For this review, use the dimensioned drawing (mm, ordinates from the lowest corner) and the shaded views. A direction names the side the tool comes from. Round coordinates to 2 decimals unless told otherwise and drop trailing zeros. Loops run counter-clockwise (first coordinate to the right, second up) from the corner with the lowest first, then second, coordinate; pieces in that order, holes last. Notation, with made-up numbers: M 65,44 L 100,44 A8 ccw 100,56 Z; hole C 31.25,-36.75 d8. An arc over 180 degrees is marked long. Answer as a JSON object with one key per item and string values. Group by question number.
Item 1: Consider section A-A (x = 21.5). Give the boundary of the cut face in (y, z), and give its area (3 significant figures).
Item 2: Tool access review of the marked faces 5 and 6: name each direction out of +Z, -Z, +X, -X, +Y, -Y from which nothing blocks a thin tool from reaching the whole face with its end or side.
Item 3: To check wall thickness, follow line 1 (X direction, y = 5.25, z = 36); line 2 (X direction, y = 9, z = 21.5); line 3 (X direction, y = 8.5, z = 35). State the ranges of each line that lie inside material, in increasing order.
Item 4: Consider section B-B (z = 28). Give the boundary of the cut face in (x, y).
Item 5: The part is to be moulded in two halves that separate along X. For the marked faces 1, 2, 3 and 4, say which applies: +X half, -X half, draft (parallel to the pull), parting line (faces both ways), or undercut.
Item 6: Insertion check: P1, Ø4, axis at x = 4, z = 36, coming from the +Y side. The pin has a flat end and moves straight along its axis. Give the tip position at first contact, or say it passes through.
Item 7: Consider section D-D (x = 36). Give the boundary of the cut face in (y, z), and give its area (3 significant figures).
Item 8: Consider section C-C (y = 11.5). Give the boundary of the cut face in (x, z).
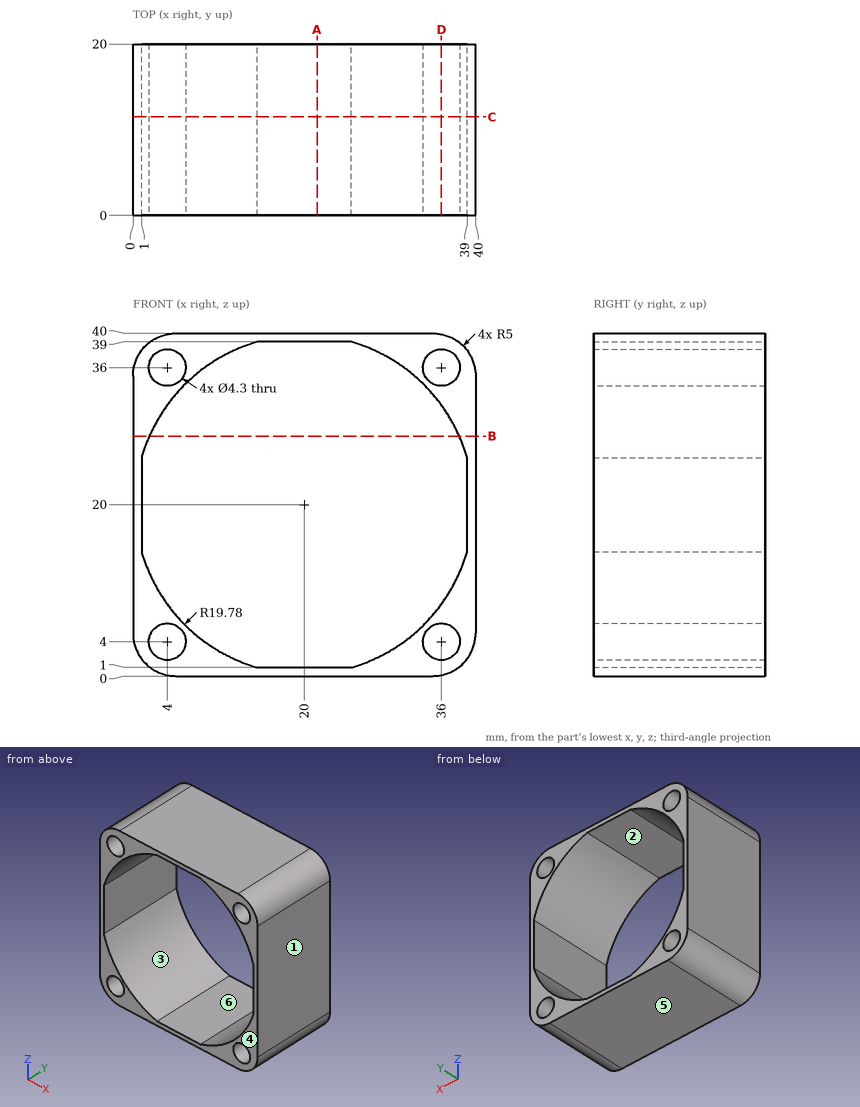
Geometry results:
{
 "1": {"outline": "M 0,0 L 20,0 L 20,1 L 0,1 Z; M 0,39 L 20,39 L 20,40 L 0,40 Z", "area": "40.0 mm^2"},
 "2": {"face 5": "-Z, +X, -X, +Y, -Y", "face 6": "+Y, -Y"},
 "3": {"line 1": "x = 0.1 to 1.85, 6.15 to 8.37, 31.63 to 33.85, 38.15 to 39.9", "line 2": "x = 0 to 1, 39 to 40", "line 3": "x = 0 to 2.1, 5.9 to 7.11, 32.89 to 34.1, 37.9 to 40"},
 "4": {"outline": "M 0,0 L 1.91,0 L 1.91,20 L 0,20 Z; M 38.09,0 L 40,0 L 40,20 L 38.09,20 Z"},
 "5": {"face 1": "+X half", "face 2": "undercut", "face 3": "undercut", "face 4": "draft"},
 "6": {"P1": "passes through"},
 "7": {"outline": "M 0,0.1 L 20,0.1 L 20,1.85 L 0,1.85 Z; M 0,6.15 L 20,6.15 L 20,8.37 L 0,8.37 Z; M 0,31.63 L 20,31.63 L 20,33.85 L 0,33.85 Z; M 0,38.15 L 20,38.15 L 20,39.9 L 0,39.9 Z", "area": "159 mm^2"},
 "8": {"outline": "M 0,5 A5 ccw 5,0 L 35,0 A5 ccw 40,5 L 40,35 A5 ccw 35,40 L 5,40 A5 ccw 0,35 Z; hole M 1,14.5 A19.78 ccw 14.5,1 L 25.5,1 A19.78 ccw 39,14.5 L 39,25.5 A19.78 ccw 25.5,39 L 14.5,39 A19.78 ccw 1,25.5 Z; hole C 4,4 d4.3; hole C 4,36 d4.3; hole C 36,4 d4.3; hole C 36,36 d4.3"}
}
